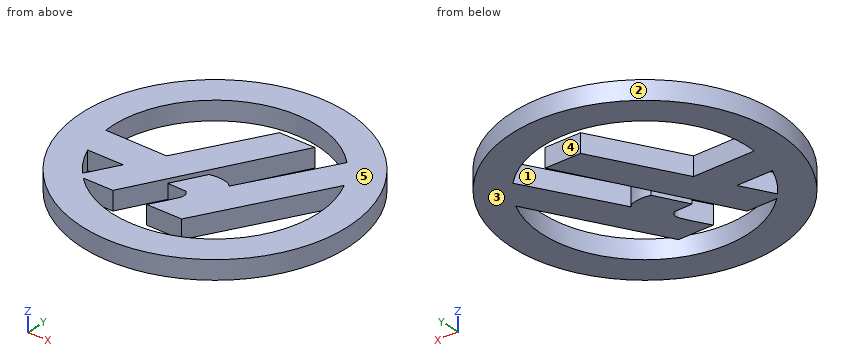
from build123d import *

# Parameters (mm, degrees)
SKETCH1_R           = 354.154198638
BOSS_EXTRUDE4_DEPTH = 50


with BuildPart() as part:
    # Sketch1 → Boss-Extrude4 (new body)
    with BuildSketch(Plane.XY):
        with Locations((456.634031844, 370.797239723)):
            Circle(SKETCH1_R)
        with BuildLine():
            Line((652.184505988, 561.696856288), (520, 338))
            add(Edge.make_bspline(
                [(520, 338), (516, 341), (512.856486558, 345.810656353), (508, 347), (483.294181497, 353.050404531), (477.851743634, 351.141957272), (459, 348)],
                knots=[0, 0, 0, 0, 1, 1, 1, 2, 2, 2, 2], degree=3))
            Line((459, 348), (414.15311107, 268.000000001))
            Line((414.15311107, 268.000000001), (463, 267))
            add(Edge.make_bspline(
                [(463, 267), (465.333333333, 263.666666667), (469.050440025, 260.956499894), (470, 257), (471.16945492, 252.127271165), (471.128314939, 246.536671316), (469, 242), (458.288028235, 219.166586501), (444.333333333, 198), (432, 176)],
                knots=[0, 0, 0, 0, 1, 1, 1, 2, 2, 2, 3, 3, 3, 3], degree=3))
            Line((432, 176), (523.783724069, 176))
            Line((523.783724069, 176), (703.607534398, 487.787583679))
            ThreePointArc((703.607534398, 487.787583679), (614.979125151, 148.065376335), (264.996930573, 175.96943637))
            Line((264.996930573, 175.96943637), (342.999405137, 176))
            Line((342.999405137, 176), (562.999999995, 567.000000012))
            Line((562.999999995, 567.000000012), (470.080751257, 567.000000012))
            Line((470.080751257, 567.000000012), (344.999999995, 351.000000012))
            Line((344.999999995, 351.000000012), (183.999999995, 352.000000012))
            ThreePointArc((183.999999995, 352.000000012), (344.926101955, 620.204516968), (652.184505988, 561.696856288))
        make_face(mode=Mode.SUBTRACT)
        with BuildLine():
            Line((203.423883848, 268.000000001), (297, 268.000000001))
            Line((297, 268.000000001), (251.884299831, 189.799453042))
            ThreePointArc((251.884299831, 189.799453042), (224.339726467, 226.845833922), (203.423883848, 268.000000001))
        make_face(mode=Mode.SUBTRACT)
    extrude(amount=BOSS_EXTRUDE4_DEPTH)


solid = part.part
Here's how the part is built. I have some questions about the finished solid (model axes, mm). Face numbers are marked on the shaded views. A direction names the side the tool comes from. Coordinates: 2 decimals unless noted, no trailing zeros. Loops run counter-clockwise (first coordinate to the right, second up) from the corner with the lowest first, then second, coordinate; pieces in that order, holes last.
1. Imagine slicing it at B-B, the plane y = 512. Please give me the cut outline in (x, z).
2. Imagine slicing it at C-C, the plane y = 119.5. Please give me the cut outline in (x, z).
3. Imagine slicing it at A-A, the plane x = 636.5. Please give me the cut outline in (y, z).
4. If we mould it in two halves opening along X, with no side actions, what happens to the marked faces 1, 2 and 3? For each: pulls with the +X half, pulls with the -X half, needs draft (parallel to the pull), parting line crosses it, or undercut.
5. Imagine slicing it at D-D, the plane x = 278.5. Please give me the cut outline in (y, z).
6. For the marked faces 4 and 5, which set-ups out of +Z, -Z, +X, -X, +Y, -Y let a thin tool reach every point of the face, with its end or its side?
7. For P1, Ø10, axis at y = 404.5, z = 35, coming from the +X side; P2, Ø2, axis at x = 637.5, z = 43, coming from the +Y side; P3, Ø2, axis at y = 412.5, z = 16, coming from the +X side, each with a flat end and sliding along its axis, tell me the tip position at first contact or that it passes through.
8. I need wall thicknesses on L1, parallel to Y at x = 428, z = 47; L2, parallel to Y at x = 317.5, z = 10.5; L3, parallel to Y at x = 427, z = 9. Which ranges of each line are inside material? Lowest first, please.
Taken from the geometry:
1. outline: (131.85, 0) - (222.66, 0) - (222.66, 50) - (131.85, 50) - close; (438.23, 0) - (532.05, 0) - (532.05, 50) - (438.23, 50) - close; (622.82, 0) - (781.42, 0) - (781.42, 50) - (622.82, 50) - close
2. outline: (207.08, 0) - (349.25, 0) - (349.25, 50) - (207.08, 50) - close; (564.02, 0) - (706.18, 0) - (706.18, 50) - (564.02, 50) - close
3. outline: (65.72, 0) - (165.05, 0) - (165.05, 50) - (65.72, 50) - close; (371.43, 0) - (535.15, 0) - (535.15, 50) - (371.43, 50) - close; (576.54, 0) - (675.88, 0) - (675.88, 50) - (576.54, 50) - close
4. face 1: undercut
4. face 2: parting line crosses it
4. face 3: needs draft
5. outline: (64.7, 0) - (163.55, 0) - (163.55, 50) - (64.7, 50) - close; (175.97, 0) - (235.93, 0) - (235.93, 50) - (175.97, 50) - close; (268, 0) - (351.41, 0) - (351.41, 50) - (268, 50) - close; (578.04, 0) - (676.89, 0) - (676.89, 50) - (578.04, 50) - close
6. face 4: +Z, -Z
6. face 5: +Z, +X, -X, +Y, -Y
7. P1: stops at x = 809.62
7. P2: stops at y = 675.88
7. P3: stops at x = 808.44
8. L1: y = 17.8 to 99.02, 267.72 to 292.7, 327.07 to 494.33, 642.57 to 723.79
8. L2: y = 45.12 to 135.59, 175.99 to 351.17, 606.01 to 696.48
8. L3: y = 17.89 to 99.13, 267.74 to 290.92, 325.29 to 492.6, 642.47 to 723.71
